For this review, take the finished solid that the model builds, in its own axes (mm). Face numbers are marked on the shaded views. A direction names the side the tool comes from. Coordinates: 2 decimals unless noted, no trailing zeros. Write each loop counter-clockwise with the first axis right and the second up, starting at its lowest first coordinate (ties: lowest second). Pieces come first, ordered by that corner, then holes. Notation, with made-up numbers: (-1, 7) - (14, 7) arc R18 cw to (14, 26) - close; hole circle Ø6 at (88, 23). An arc over 180 degrees is marked (long way). Use one line per item in the form item = value. Start each with the question number.
1) We need section B-B (y = 5.75). Give the boundary of the cut face in (x, z).
2) We need section D-D (x = -197). Give the boundary of the cut face in (y, z), plus the area to 3 significant figures.
3) We need section A-A (z = -16). Give the boundary of the cut face in (x, y).
4) We need section C-C (z = -25.5). Give the boundary of the cut face in (x, y), plus the area to 3 significant figures.
5) For L1, parallel to Z at x = -193, y = 4.5; L2, parallel to X at y = 4.75, z = -18; L3, parallel to Z at x = -193.25, y = 9.25, list the stretches that pass through material, from the lowest coordinate up. Write a range as from..to.
6) Insertion check: P1, Ø1.5, axis at x = -192, z = 24, coming from the +Y side; P2, Ø4, axis at x = -192.5, y = 8.5, coming from the +Z side; P3, Ø2, axis at x = -201, y = 4.5, coming from the +Z side. Each pin has a flat end and moves straight along its axis. Give the tip position at first contact, or say it passes through.
7) Mouldability with a two-part tool opening along Z and no side actions: class the marked faces 3, 4 and 5 as pulls with the +Z half, pulls with the -Z half, needs draft (parallel to the pull), parting line crosses it, or undercut.
8) Tool access review of the marked faces 1 and 2: name each direction out of +Z, -Z, +X, -X, +Y, -Y from which nothing blocks a thin tool from reaching the whole face with its end or side.
```python
from build123d import *

# Parameters (mm, degrees)
BOSS_EXTRUDE1_DEPTH        = 10
CUT_EXTRUDE1_DEPTH         = 5
FILLET1_R                  = 2
CUT_EXTRUDE2_START         = -2.5
CUT_EXTRUDE2_DEPTH         = 2.5
F_3_1_3_1_DIAMETER_HOLE1_D = 3.1


with BuildPart() as part:
    # Sketch1 → Boss-Extrude1 (new body)
    with BuildSketch(Plane(origin=(0, 0, 0), x_dir=(1, 0, 0), z_dir=(0, 1, 0))):
        with BuildLine():
            ThreePointArc((-187.660784713, 29.722548358), (-190, 0), (-187.660784713, -29.722548358))
            Line((-187.660784713, -29.722548358), (-197.537668119, -31.286893008))
            ThreePointArc((-197.537668119, -31.286893008), (-200, 0), (-197.537668119, 31.286893008))
            Line((-197.537668119, 31.286893008), (-187.660784713, 29.722548358))
        make_face()
        with BuildLine():
            ThreePointArc((-197.537668119, -31.286893008), (-200, 0), (-197.537668119, 31.286893008))
            Line((-197.537668119, 31.286893008), (-200.500733141, 31.756196403))
            ThreePointArc((-200.500733141, 31.756196403), (-203, 0), (-200.500733141, -31.756196403))
            Line((-200.500733141, -31.756196403), (-197.537668119, -31.286893008))
        make_face()
        with BuildLine():
            Line((-184.697719691, 29.253244963), (-187.660784713, 29.722548358))
            ThreePointArc((-187.660784713, 29.722548358), (-190, 0), (-187.660784713, -29.722548358))
            Line((-187.660784713, -29.722548358), (-184.697719691, -29.253244963))
            ThreePointArc((-184.697719691, -29.253244963), (-187, 0), (-184.697719691, 29.253244963))
        make_face()
    extrude(amount=BOSS_EXTRUDE1_DEPTH)

    # Sketch15 → Cut-Extrude1 (cut)
    with BuildSketch(Plane(origin=(0, 10, 0), x_dir=(1, 0, 0), z_dir=(0, 1, 0))):
        with BuildLine():
            Line((-199.749843554, 10), (-189.73665961, 10))
            ThreePointArc((-189.73665961, 10), (-188.956218405, 19.88837666), (-187.660784713, 29.722548358))
            Line((-187.660784713, 29.722548358), (-197.537668119, 31.286893008))
            ThreePointArc((-197.537668119, 31.286893008), (-198.928692466, 20.673057674), (-199.749843554, 10))
        make_face()
        with BuildLine():
            ThreePointArc((-187.660784713, -29.722548358), (-188.956218405, -19.88837666), (-189.73665961, -10))
            Line((-189.73665961, -10), (-199.749843554, -10))
            ThreePointArc((-199.749843554, -10), (-198.928692466, -20.673057674), (-197.537668119, -31.286893008))
            Line((-197.537668119, -31.286893008), (-187.660784713, -29.722548358))
        make_face()
    extrude(amount=-CUT_EXTRUDE1_DEPTH, mode=Mode.SUBTRACT)

    # Fillet1
    fillet1_edges = [part.edges().sort_by_distance(p)[0] for p in [
        (-200.500733141, 5, 31.756196403),
        (-200.500733141, 5, -31.756196403),
        (-184.697719691, 5, -29.253244963),
        (-184.697719691, 5, 29.253244963),
    ]]
    fillet(fillet1_edges, radius=FILLET1_R)

    # Sketch19 → Cut-Extrude2 (cut)
    with BuildSketch(Plane.XZ.offset(CUT_EXTRUDE2_START)):
        with BuildLine():
            Line((-198.515528472, -31.441770873), (-186.662644351, -29.564458455))
            ThreePointArc((-186.662644351, -29.564458455), (-185.363721979, -28.773196969), (-184.996936421, -27.297133819))
            ThreePointArc((-184.996936421, -27.297133819), (-187, 0), (-184.996936421, 27.297133819))
            ThreePointArc((-184.996936421, 27.297133819), (-185.363721979, 28.773196969), (-186.662644351, 29.564458455))
            Line((-186.662644351, 29.564458455), (-198.515528472, 31.441770873))
            ThreePointArc((-198.515528472, 31.441770873), (-200.012003377, 31.078559473), (-200.806789416, 29.759592144))
            ThreePointArc((-200.806789416, 29.759592144), (-203, 0), (-200.806789416, -29.759592144))
            ThreePointArc((-200.806789416, -29.759592144), (-200.012003377, -31.078559473), (-198.515528472, -31.441770873))
        make_face()
    extrude(amount=CUT_EXTRUDE2_DEPTH, mode=Mode.SUBTRACT)

    # Ø3.1 (3.1) Diameter Hole1 (through all)
    with Locations(Plane(origin=(0, 2.5, 0), x_dir=(-1, 0, 0), z_dir=(0, -1, 0))):
        with Locations((194.257966128, 16.995369836), (194.257966128, -16.995369836)):
            Hole(F_3_1_3_1_DIAMETER_HOLE1_D / 2)


solid = part.part
```
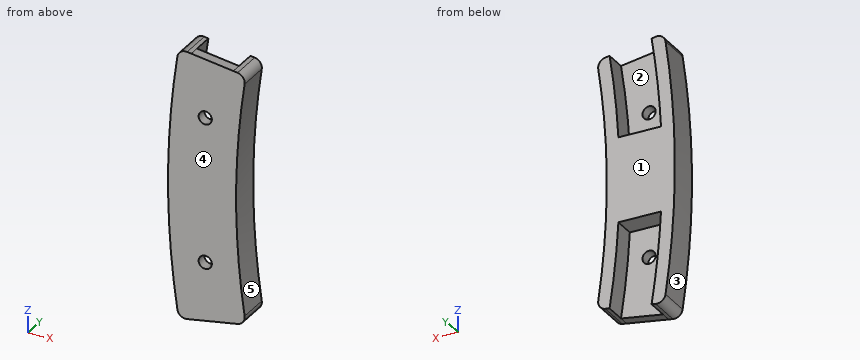
Determined:
q1.outline = (-200.81, -29.76) arc R2 ccw to (-198.52, -31.44) - (-197.54, -31.29) arc R200 cw to (-199.75, -10) - (-189.74, -10) arc R190 ccw to (-187.66, -29.72) - (-186.66, -29.56) arc R2 ccw to (-185, -27.3) arc R187 cw to (-185, 27.3) arc R2 ccw to (-186.66, 29.56) - (-187.66, 29.72) arc R190 ccw to (-189.74, 10) - (-199.75, 10) arc R200 cw to (-197.54, 31.29) - (-198.52, 31.44) arc R2 ccw to (-200.81, 29.76) arc R203 ccw to start
q2.outline = (2.5, -31.2) - (5, -31.2) - (5, -10) - (10, -10) - (10, 10) - (5, 10) - (5, 31.2) - (2.5, 31.2) - close
q2.area = 256 mm²
q3.outline = (-202.37, 2.5) - (-195.45, 2.5) - (-195.45, 5) - (-199.36, 5) - (-199.36, 10) - (-202.37, 10) - close; (-193.07, 2.5) - (-186.31, 2.5) - (-186.31, 10) - (-189.33, 10) - (-189.33, 5) - (-193.07, 5) - close
q4.outline = (-201.39, 2.5) - (-185.25, 2.5) - (-185.25, 10) - (-188.28, 10) - (-188.28, 5) - (-198.37, 5) - (-198.37, 10) - (-201.39, 10) - close
q4.area = 70.6 mm²
q5.L1 = -30.57..-17.9, -16.09..16.09, 17.9..30.57
q5.L2 = -202.2..-195.44, -193.08..-186.13
q5.L3 = -10..10
q6.P1 = 5
q6.P2 = 10
q6.P3 = 31.09
q7.face_3 = parting line crosses it
q7.face_4 = needs draft
q7.face_5 = undercut
q8.face_1 = +Z, -Z, +X, -X, +Y
q8.face_2 = +Y
